from build123d import *

# Parameters (mm, degrees)
SKETCH1_W           = 12.5
SKETCH1_H           = 7
BOSS_EXTRUDE1_DEPTH = 9.25
SKETCH2_W           = 12.5
SKETCH2_H           = 7
BOSS_EXTRUDE2_DEPTH = 0.5


with BuildPart() as part:
    # Sketch1 → Boss-Extrude1 (new body)
    with BuildSketch(Plane(origin=(0, 0, 0), x_dir=(1, 0, 0), z_dir=(0, 1, 0))):
        with Locations((0, 3.5)):
            Rectangle(SKETCH1_W, SKETCH1_H)
        Polygon((-5.75, 5.25), (-5.75, 0.75), (-2.25, 0.75), (-2.25, 5.25), (-3.05, 5.25), (-3.05, 5.65), (-2.25, 6.5), (-5.75, 6.5), (-4.95, 5.65), (-4.95, 5.25), align=None, mode=Mode.SUBTRACT)
        Polygon((-1.75, 5.25), (-1.75, 0.75), (1.75, 0.75), (1.75, 5.25), (0.95, 5.25), (0.95, 5.65), (1.75, 6.5), (-1.75, 6.5), (-0.95, 5.65), (-0.95, 5.25), align=None, mode=Mode.SUBTRACT)
        Polygon((2.25, 5.25), (2.25, 0.75), (5.75, 0.75), (5.75, 5.25), (4.95, 5.25), (4.95, 5.65), (5.75, 6.5), (2.25, 6.5), (3.05, 5.65), (3.05, 5.25), align=None, mode=Mode.SUBTRACT)
    extrude(amount=BOSS_EXTRUDE1_DEPTH)

    # Sketch2 → Boss-Extrude2 (add)
    with BuildSketch(Plane.XZ):
        with Locations((0, -3.5)):
            Rectangle(SKETCH2_W, SKETCH2_H)
    extrude(amount=BOSS_EXTRUDE2_DEPTH)


solid = part.part
Check sheet for the modelled part. Datum: model origin and axes. Units: mm. A direction names the side the tool comes from. Round coordinates to 2 decimals unless told otherwise and drop trailing zeros. Loops run counter-clockwise (first coordinate to the right, second up) from the corner with the lowest first, then second, coordinate; pieces in that order, holes last. Notation, with made-up numbers: M -17.5,69 L 11.5,69 A30 ccw 11.5,92 Z; hole C 54,89.25 d2. An arc over 180 degrees is marked long. One line per question, with ' | ' between items. Start each with the question number.
Item 1: Section check A-A (y = 6.5). State how many separate pieces and enclosed holes the cut face has, and give its area (3 significant figures).
Item 2: Scan lines: probe 1 along X at (y, z) = (8.25, -4.25); probe 2 along Z at (x, y) = (-3.25, 6.5); probe 3 along Z at (x, y) = (-1.5, 9). Record each from-to range of solid material in increasing order.
Item 3: Gauge pin test, flat ends, axial feed: pin 1 Ø3 at (x, y) = (-4.5, 5) entering from +Z; pin 2 Ø3 at (x, z) = (4, -2.5) entering from +Y. Record the tip position at first contact, or that the pin passes through.
Item 4: Section check B-B (z = -4). Record the boundary of the cut face in (x, y), and give its area (4 significant figures).
Item 5: Set-up check for faces 4 (the face through (-6.25, 4, -4)), 5 (the face through (0, 5, -0.75)): record each of +Z, -Z, +X, -X, +Y, -Y from which the full face is reachable in a straight line by a thin tool's end or side.
Item 6: Release check for a two-part mould opening along X. For faces 1 (the face through (6.25, 4, -4)), 2 (the face through (0, 4, -7)), 3 (the face through (-4, 0, -4)) record: released by +X, released by -X, zero draft, split by the parting line, or undercut.
Item 7: Section check C-C (x = 4.5). Record the boundary of the cut face in (y, z).
Item 8: Section check D-D (x = -5.5). Record the boundary of the cut face in (y, z).
Worked out:
1) separate pieces: 1 | enclosed holes: 3 | area: 31.1 mm^2
2) probe 1: -6.25 to -5.75, -2.25 to -1.75, 1.75 to 2.25, 5.75 to 6.25 | probe 2: -7 to -6.5, -0.75 to 0 | probe 3: -7 to -6.5, -6.23 to -5.25, -0.75 to 0
3) pin 1: z = 0 | pin 2: y = 0
4) outline: M -6.25,-0.5 L 6.25,-0.5 L 6.25,9.25 L 5.75,9.25 L 5.75,0 L 2.25,0 L 2.25,9.25 L 1.75,9.25 L 1.75,0 L -1.75,0 L -1.75,9.25 L -2.25,9.25 L -2.25,0 L -5.75,0 L -5.75,9.25 L -6.25,9.25 Z | area: 24.75 mm^2
5) face 4: +Z, -Z, -X, +Y, -Y | face 5: +Y
6) face 1: released by +X | face 2: zero draft | face 3: undercut
7) outline: M -0.5,-7 L 9.25,-7 L 9.25,-6.5 L 0,-6.5 L 0,-0.75 L 9.25,-0.75 L 9.25,0 L -0.5,0 Z
8) outline: M -0.5,-7 L 9.25,-7 L 9.25,-6.5 L 0,-6.5 L 0,-6.23 L 9.25,-6.23 L 9.25,-5.25 L 0,-5.25 L 0,-0.75 L 9.25,-0.75 L 9.25,0 L -0.5,0 Z
